Build history of the part. All positions in model axes, mm. A direction names the side the tool comes from. Give positions to 0.01 mm unless a question says otherwise; leave off trailing zeros. Loops run counter-clockwise (first coordinate to the right, second up) from the corner with the lowest first, then second, coordinate; pieces in that order, holes last. Notation, with made-up numbers: (35, 26) -> (55, 26) arc R13 cw to (55, 44) -> close; hole circle Ø3 at (48, -18.75). An arc over 180 degrees is marked (long way). Answer as a JSON object with one key per item and string values. Group by question number.
Autodesk Inventor part; units mm, degrees
ref_plane "YZ Plane" through (0, 0, 0) normal (1, 0, 0) x (0, 1, 0)
ref_plane "XZ Plane" through (0, 0, 0) normal (0, 1, 0) x (-1, 0, 0)
ref_plane "XY Plane" through (0, 0, 0) normal (0, 0, 1) x (1, 0, 0)
sketch "Sketch1" plane through (0, 0, 0) normal (0, 1, 0) x (-1, 0, 0)
  line L0 (0, 0) -> (0, 1200)
  line L1 (0, 1200) -> (240, 1200)
  line L2 (370, 400) -> (570, 400)
  line L3 (240, 1200) -> (370, 400)
  line L4 (570, 400) -> (570, 250)
  line L5 (570, 250) -> (370, 250)
  line L6 (370, 0) -> (370, 250)
  line L7 (370, 0) -> (280, 0)
  line L8 (280, 0) -> (280, 90)
  line L9 (280, 90) -> (90, 90)
  line L10 (90, 90) -> (90, 0)
  line L11 (90, 0) -> (0, 0)
  dimension "d2" = 1200
  dimension "d4" = 200
  dimension "d8" = 370
  dimension "d9" = 150
  dimension "d10" = 250
  dimension "d11" = 90
  dimension "d12" = 90
  dimension "d13" = 190
  dimension "d14" = 240
extrude "Extrusion1" add sketch "Sketch1" along normal blind 20
sketch "Sketch2" plane through (0, 0, 0) normal (0, -1, 0) x (1, 0, 0)
  line L0 (0, 0) -> (0, 1200)
  line L1 (0, 1200) -> (-240, 1200)
  line L2 (-240, 1200) -> (-240, 400)
  line L3 (-370, 400) -> (-570, 400)
  line L4 (-570, 400) -> (-570, 0)
  line L5 (-570, 0) -> (0, 0)
sketch "Sketch3" plane through (0, 0, 0) normal (0, -1, 0) x (1, 0, 0)
  line L0 (0, 0) -> (0, 1200)
  line L1 (0, 1200) -> (-240, 1200)
  line L2 (-240, 1200) -> (-370, 400)
  line L3 (-370, 400) -> (-570, 400)
  line L4 (-570, 400) -> (-570, 250)
  line L5 (-570, 250) -> (-370, 250)
  line L6 (-370, 250) -> (-370, 0)
  line L7 (-370, 0) -> (-280, 0)
  line L8 (-280, 0) -> (-280, 90)
  line L9 (-280, 90) -> (-90, 90)
  line L10 (-90, 90) -> (-90, 0)
  line L11 (-90, 0) -> (0, 0)
sketch "Sketch4" plane through (0, 0, 0) normal (0, -1, 0) x (1, 0, 0)
  line L0 (0, 0) -> (0, 1200)
  line L1 (0, 1200) -> (-240, 1200)
  line L2 (0, 0) -> (-8, 0)
  line L3 (-8, 0) -> (-8, 1200)
  line L4 (-8, 1200) -> (0, 1200)
  line L5 (0, 1200) -> (0, 0)
  dimension "d15" = 8
extrude "Extrusion2" cut sketch "Sketch4" against normal blind 10
properties part number "seitenteil"
(1) Saw through at B-B on z = 140.5. List the corners of the cut face in (x, y).
(2) Probe line 1 along X through (y, z) = (18.75, 209); line 2 along Z through (x, y) = (-512.5, 8.25); line 3 along Z through (x, y) = (-226, 3.25). List the from-to ranges inside material, lowest first. Write a range as [from, to].
(3) Saw through at C-C on x = -485. List the corners of the cut face in (y, z).
(4) Saw through at D-D on z = 886.5. List the corners of the cut face in (x, y), plus the area to 3 significant figures.
(5) Saw through at A-A on y = 5.75. List the corners of the cut face in (x, z).
(6) Pin check, flat tips, straight feed: pin 1 (12 mm diameter, centred on y = 14.5, z = 984.5, fed in from -X); pin 2 (10 mm diameter, centred on x = -186.5, y = 12, fed in from -Z); pin 3 (2 mm diameter, centred on y = 6.5, z = 1078.5, fed in from +X). Stop position of each tip, or through.
(7) 3-axis set-ups, long thin cutter, end or side, ignore diameter. For faces 4 (the flat face through (-280, 10, 44)), 5 (the flat face through (-469, 10, 400)), 6 (the flat face through (-118, 10, 1200)), 7 (the flat face through (-471, 10, 250)), 8 (the flat face through (-46, 10, 0)): which of +Z, -Z, +X, -X, +Y, -Y reach the whole face in a straight line?
(8) Pull direction X, two halves, no side cores. Call faces 1 (the flat face through (-186, 10, 90)), 2 (the flat face through (-154, 20, 608)), 3 (the flat face through (-370, 10, 123)): pulls with the +X half, pulls with the -X half, needs draft (parallel to the pull), parting line crosses it, or undercut.
Calculated:
{
 "1": {"outline": "(-370, 0) -> (-8, 0) -> (-8, 10) -> (0, 10) -> (0, 20) -> (-370, 20) -> close"},
 "2": {"line 1": "x = [-370, 0]", "line 2": "z = [250, 400]", "line 3": "z = [90, 1200]"},
 "3": {"outline": "(0, 250) -> (20, 250) -> (20, 400) -> (0, 400) -> close"},
 "4": {"outline": "(-290.94, 0) -> (-8, 0) -> (-8, 10) -> (0, 10) -> (0, 20) -> (-290.94, 20) -> close", "area": "5,740 mm^2"},
 "5": {"outline": "(-570, 250) -> (-370, 250) -> (-370, 0) -> (-280, 0) -> (-280, 90) -> (-90, 90) -> (-90, 0) -> (-8, 0) -> (-8, 1200) -> (-240, 1200) -> (-370, 400) -> (-570, 400) -> close"},
 "6": {"pin 1": "stops at x = -275.99", "pin 2": "stops at z = 90", "pin 3": "stops at x = -8"},
 "7": {"face 4": "-Z, +Y, -Y", "face 5": "+Z, -X, +Y, -Y", "face 6": "+Z, +X, -X, +Y, -Y", "face 7": "-Z, -X, +Y, -Y", "face 8": "-Z, +X, -X, +Y, -Y"},
 "8": {"face 1": "undercut", "face 2": "needs draft", "face 3": "pulls with the -X half"}
}
